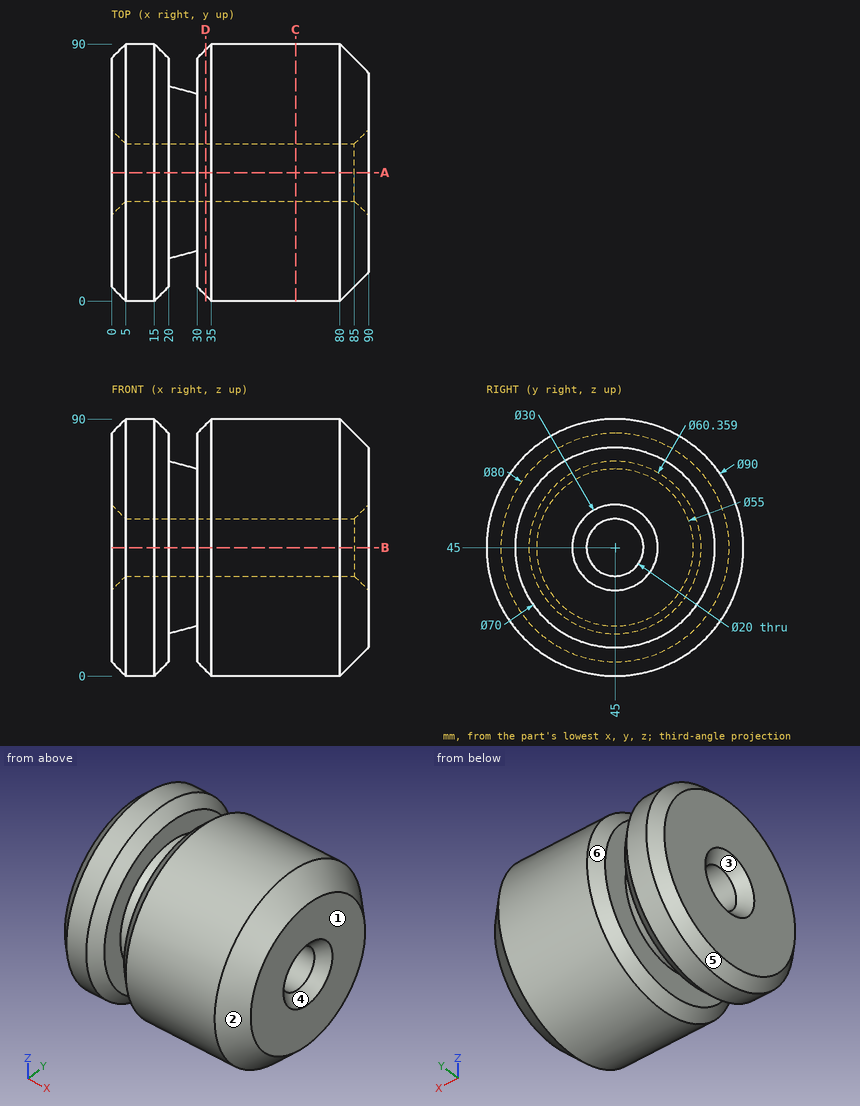
Study the drawing (mm; zero at the part's minimum x, y, z) and answer. A direction names the side the tool comes from. Round coordinates to 2 decimals unless told otherwise and drop trailing zeros. Order: outer loops, then holes, each group sorted by start corner. A loop starts at its lowest first (then second) coordinate and runs counter-clockwise, first axis right, second up. Notation, with made-up numbers: (-28, -11.75) -> (12, -11.75) arc R16 ccw to (12, -0.75) -> close; hole circle Ø11 at (-38.5, -35.75). An arc over 180 degrees is marked (long way). Answer as CSV lines item,"result". Start each with the question number.
(1) A tool of negligible diameter and unlimited length cuts with its end or side. For the marked faces 5 and 6, from which of +Z, -Z, +X, -X, +Y, -Y can it reach the whole face along a straight path? Write none if from no direction.
(2) The part is cut by section D-D (x = 33). Determine the outline of the cut face in (y, z).
(3) Flat-ended cylindrical pins translate along their axes: pin 1 Ø1.5 at (x, z) = (30, 14) entering from -Y; pin 2 Ø1.5 at (x, y) = (14.5, 19.5) entering from +Z; pin 3 Ø2 at (x, y) = (40.5, 74) entering from -Z. Find the tip coordinate at first contact, or state that the pin passes through.
(4) The part is cut by section C-C (x = 64.5). Determine the outline of the cut face in (y, z).
(5) For a pull along Z with two mould halves and no side action, classify the marked faces 1, 2, 3 and 4 as +Z half, -Z half, draft (parallel to the pull), parting line (faces both ways), or undercut.
(6) Find the intervals of material crossed by probe 1 along Z at (x, y) = (54, 45); probe 2 along Z at (x, y) = (34.5, 38), in increasing order. Write a range as from..to.
(7) The part is cut by section A-A (y = 45). Determine the outline of the cut face in (x, z).
Evaluation:
1,face 5,"-X"
1,face 6,"none"
2,outline,"circle Ø86 at (45, 45); hole circle Ø20 at (45, 45)"
3,pin 1,"y = 18.26"
3,pin 2,"z = 82.58"
3,pin 3,"z = 9.77"
4,outline,"circle Ø90 at (45, 45); hole circle Ø20 at (45, 45)"
5,face 1,"draft"
5,face 2,"parting line"
5,face 3,"undercut"
5,face 4,"undercut"
6,probe 1,"0..35, 55..90"
6,probe 2,"1.05..37.86, 52.14..88.95"
7,outline,"(0, 5) -> (5, 0) -> (15, 0) -> (20, 5) -> (20, 14.82) -> (30, 17.5) -> (30, 5) -> (35, 0) -> (80, 0) -> (90, 10) -> (90, 30) -> (85, 35) -> (5, 35) -> (0, 30) -> close; (0, 60) -> (5, 55) -> (85, 55) -> (90, 60) -> (90, 80) -> (80, 90) -> (35, 90) -> (30, 85) -> (30, 72.5) -> (20, 75.18) -> (20, 85) -> (15, 90) -> (5, 90) -> (0, 85) -> close"
